CAD build for the part. Positions are in the model's coordinates, mm. Face numbers are marked on the shaded views. Coordinates: 2 decimals unless noted, no trailing zeros. Order: outer loops, then holes, each group sorted by start corner. A loop starts at its lowest first (then second) coordinate and runs counter-clockwise, first axis right, second up.
from build123d import *

# Parameters (mm, degrees)
F0_W     = 152.4
F0_H     = 54.999991
F1_DEPTH = 10.2616
F2_W     = 4.790508
F2_H     = 12.7
F2_H_2   = 7.501991
F3_DEPTH = 7.9248
F5_R     = 1.4986
F6_DEPTH = 6.35
F4_R     = 1.4986
F7_DEPTH = 6.35


with BuildPart() as f1:
    # F0 (on Top) → F1 (new body)
    with BuildSketch(Plane.XY):
        with Locations((14.24603, 4.996552)):
            Rectangle(F0_W, F0_H)
    extrude(amount=F1_DEPTH)

    # F2 (on face) → F3 (cut)
    with BuildSketch(Plane.XY.offset(10.2616)):
        Polygon((-57.25497, 27.797548), (-57.25497, -17.804443), (-19.15497, 6.281104), align=None)
        Polygon((0.392403, 27.797548), (-47.199331, 27.797548), (-19.15497, 11.959886), (-14.07497, 11.959886), align=None)
        Polygon((-19.15497, 0), (-47.199331, -17.804443), (0.392403, -17.804443), (-14.07497, 0), align=None)
        Polygon((5.496245, 27.797548), (-14.07497, 6.281104), (5.496245, -17.804443), align=None)
        with Locations((11.848874, 21.447548)):
            Rectangle(F2_W, F2_H)
        with Locations((11.848874, 4.996552)):
            Rectangle(F2_W, F2_H_2)
        with Locations((11.848874, -11.454443)):
            Rectangle(F2_W, F2_H)
        Polygon((18.196245, -17.804443), (37.780095, 6.281104), (18.196245, 27.797548), align=None)
        Polygon((23.825141, -17.804443), (76.312438, -17.804443), (42.860095, 0), (37.780095, 0), align=None)
        Polygon((85.74703, 27.797548), (42.860095, 6.281104), (85.74703, -17.804443), align=None)
        Polygon((42.860095, 12.465476), (76.312438, 27.797548), (23.825141, 27.797548), (37.780095, 12.465476), align=None)
    extrude(amount=-F3_DEPTH, mode=Mode.SUBTRACT)

    # F5 (on face) → F6 (cut)
    with BuildSketch(Plane.YZ.offset(90.44603)):
        with Locations((19.997208, 5.1308)):
            Circle(F5_R)
        with Locations((-10.004103, 5.1308)):
            Circle(F5_R)
    extrude(amount=-F6_DEPTH, mode=Mode.SUBTRACT)

    # F4 (on face) → F7 (cut)
    with BuildSketch(Plane(origin=(-61.95397, 0, 0), x_dir=(0, -1, 0), z_dir=(-1, 0, 0))):
        with Locations((-19.997208, 5.1308)):
            Circle(F4_R)
        with Locations((10.004103, 5.1308)):
            Circle(F4_R)
    extrude(amount=-F7_DEPTH, mode=Mode.SUBTRACT)


solid = f1.part
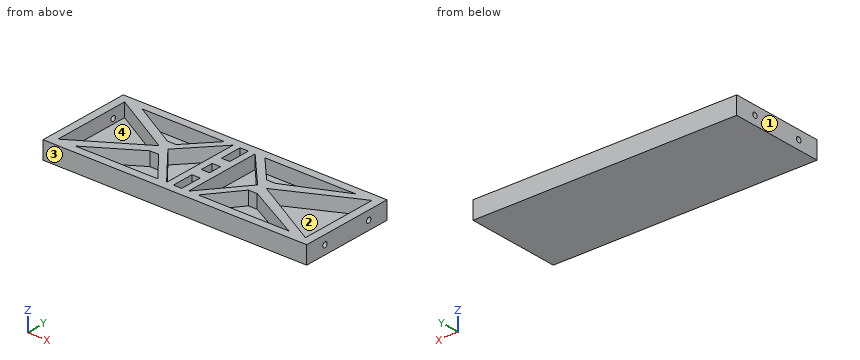
1) Pin check, flat tips, straight feed: P1, Ø2.5, axis at y = 20, z = 5.13, coming from the +X side; P2, Ø5.5, axis at x = -32.5, y = -13.5, coming from the +Z side. Stop position of each tip, or through.
2) Two-plate mould, pull along X, no slides. Class the marked faces 1, 2, 3 and 4: released by +X, released by -X, zero draft, split by the parting line, or undercut.
3) Slice it at A-A (z = 8.25). Give the number of separate pieces and of enclosed holes in the cut face, plus the area to 3 significant figures.
4) Slice it at B-B (y = -3). List the corners of the cut face in (x, z), plus the area to 3 significant figures.
5) Drill centre lines: probe 1 along Y at (x, z) = (-13, 6.25); probe 2 along Y at (x, z) = (-28.5, 8); probe 3 along X at (y, z) = (19.5, 6.5). Where is each one in solid material? Low to high.
Worked out:
1. P1: stops at x = 72.7
1. P2: stops at z = 2.34
2. face 1: released by -X
2. face 2: undercut
2. face 3: zero draft
2. face 4: undercut
3. separate pieces: 1
3. enclosed holes: 11
3. area: 3,650 mm2
4. outline: (-61.95, 0) - (90.45, 0) - (90.45, 10.26) - (85.75, 10.26) - (85.75, 2.34) - (59.39, 2.34) - (59.39, 10.26) - (48.5, 10.26) - (48.5, 2.34) - (35.43, 2.34) - (35.43, 10.26) - (30.23, 10.26) - (30.23, 2.34) - (18.2, 2.34) - (18.2, 10.26) - (5.5, 10.26) - (5.5, 2.34) - (-6.53, 2.34) - (-6.53, 10.26) - (-11.64, 10.26) - (-11.64, 2.34) - (-23.88, 2.34) - (-23.88, 10.26) - (-33.84, 10.26) - (-33.84, 2.34) - (-57.25, 2.34) - (-57.25, 10.26) - (-61.95, 10.26) - close
4. area: 778 mm2
5. probe 1: y = -22.5 to -17.8, -1.32 to 4.96, 7.46 to 13.14, 27.8 to 32.5
5. probe 2: y = -22.5 to -17.8, -5.93 to 0.37, 11.56 to 17.24, 27.8 to 32.5
5. probe 3: x = -42.56 to -32.51, -7.19 to -2.05, 5.5 to 9.45, 14.24 to 18.2, 25.75 to 31.38, 58.21 to 69.21
